CAD build for the part. Positions are in the model's coordinates, mm. Coordinates: 2 decimals unless noted, no trailing zeros. Write each loop counter-clockwise with the first axis right and the second up, starting at its lowest first coordinate (ties: lowest second). Pieces come first, ordered by that corner, then holes. Notation, with made-up numbers: (12, -35) - (42, -35) arc R20 ccw to (42, -3) - close; hole circle Ø10 at (79, 53). An arc over 180 degrees is marked (long way). One line per question, with ' | ' between items. Start each with the question number.
1. Band-saw the part on D-D, the plane x = 5. Write the cut outline in (y, z).
2. Band-saw the part on A-A, the plane y = 0. Write the cut outline in (x, z), then the cut area to 3 significant figures.
3. Two-plate mould, pull along Z, no slides. Class faces 1 (the flat face through (0, 0, 44.95)), 2 (the flat face through (0, 0, 0)), 3 (the cylindrical face through (-15.28, -11.71, 2.46)): +Z half, -Z half, draft (parallel to the pull), parting line (faces both ways), or undercut.
4. Flat gauge pins, fed straight in: P1, Ø4, axis at x = -6.5, y = 2.5, coming from the +Z side; P2, Ø6, axis at y = -5.5, z = 20.5, coming from the -X side; P3, Ø1.4, axis at x = 0.5, z = 37.5, coming from the +Y side. Where does each tip first touch, or does it go through?
5. Band-saw the part on C-C, the plane z = 41. Write the cut outline in (x, y).
6. Probe line 1 (Z direction, x = 10, y = -10.5); line 2 (Y direction, x = -16, z = 4); line 3 (X direction, y = -13, z = 3). List the from-to ranges inside material, lowest first.
7. Band-saw the part on B-B, the plane x = 0. Write the cut outline in (y, z).
from build123d import *

# Parameters (mm, degrees)
CROQUIS1_R              = 19.25
SALIENTE_EXTRUIR1_DEPTH = 5
CROQUIS2_R              = 3.5
SALIENTE_EXTRUIR2_DEPTH = 11.7
SALIENTE_EXTRUIR3_DEPTH = 28.25


with BuildPart() as part:
    # Croquis1 → Saliente-Extruir1 (new body)
    with BuildSketch(Plane.XY):
        Circle(CROQUIS1_R)
    extrude(amount=SALIENTE_EXTRUIR1_DEPTH)

    # Croquis2 → Saliente-Extruir2 (add)
    with BuildSketch(Plane.XY.offset(5)):
        Circle(CROQUIS2_R)
    extrude(amount=SALIENTE_EXTRUIR2_DEPTH)

    # Croquis3 → Saliente-Extruir3 (add)
    with BuildSketch(Plane.XY.offset(16.7)):
        with BuildLine():
            Line((-2.397394419, 2.55), (2.397394419, 2.55))
            ThreePointArc((2.397394419, 2.55), (0, -3.5), (-2.397394419, 2.55))
        make_face()
    extrude(amount=SALIENTE_EXTRUIR3_DEPTH)


solid = part.part
Filled in:
1) outline: (-18.59, 0) - (18.59, 0) - (18.59, 5) - (-18.59, 5) - close
2) outline: (-19.25, 0) - (19.25, 0) - (19.25, 5) - (3.5, 5) - (3.5, 44.95) - (-3.5, 44.95) - (-3.5, 5) - (-19.25, 5) - close | area: 472 mm²
3) face 1: +Z half | face 2: -Z half | face 3: draft
4) P1: stops at z = 5 | P2: stops at x = -2.45 | P3: stops at y = 2.55
5) outline: (-2.4, 2.55) arc R3.5 ccw (long way) to (2.4, 2.55) - close
6) line 1: z = 0 to 5 | line 2: y = -10.7 to 10.7 | line 3: x = -14.2 to 14.2
7) outline: (-19.25, 0) - (19.25, 0) - (19.25, 5) - (3.5, 5) - (3.5, 16.7) - (2.55, 16.7) - (2.55, 44.95) - (-3.5, 44.95) - (-3.5, 5) - (-19.25, 5) - close
